Build history of the part. All positions in model axes, mm. A direction names the side the tool comes from. Coordinates: 2 decimals unless noted, no trailing zeros. Write each loop counter-clockwise with the first axis right and the second up, starting at its lowest first coordinate (ties: lowest second). Pieces come first, ordered by that corner, then holes.
```python
from build123d import *

# Parameters (mm, degrees)
SKETCH_1_W          = 20
SKETCH_1_H          = 10
SKETCH_1_W_2        = 18
SKETCH_1_H_2        = 8
EXTRUDE_1_DEPTH     = 30
SKETCH_2_R          = 1.5
CUT_EXTRUDE_1_DEPTH = 20
SKETCH_3_R          = 3.5
CUT_EXTRUDE_2_DEPTH = 5


with BuildPart() as part:
    # 草图1 → 拉伸-薄壁1 (new body)
    with BuildSketch(Plane.XY):
        with Locations((19.212936099, 31.397704236)):
            Rectangle(SKETCH_1_W, SKETCH_1_H)
        with Locations((19.212936099, 31.397704236)):
            Rectangle(SKETCH_1_W_2, SKETCH_1_H_2, mode=Mode.SUBTRACT)
    extrude(amount=EXTRUDE_1_DEPTH)

    # 草图2 → 切除-拉伸1 (cut)
    with BuildSketch(Plane(origin=(29.212936099, 0, 0), x_dir=(0, 0, -1), z_dir=(1, 0, 0))):
        with Locations((-23, 31.397704236)):
            Circle(SKETCH_2_R)
        with Locations((-6, 31.397704236)):
            Circle(SKETCH_2_R)
    extrude(amount=-CUT_EXTRUDE_1_DEPTH, mode=Mode.SUBTRACT)

    # 草图3 → 切除-拉伸2 (cut)
    with BuildSketch(Plane(origin=(29.212936099, 0, 0), x_dir=(0, 0, -1), z_dir=(1, 0, 0))):
        with Locations((-23, 31.397704236)):
            Circle(SKETCH_3_R)
        with Locations((-6, 31.397704236)):
            Circle(SKETCH_3_R)
    extrude(amount=-CUT_EXTRUDE_2_DEPTH, mode=Mode.SUBTRACT)


solid = part.part
```
1. Saw through at A-A on z = 6. List the corners of the cut face in (x, y), plus the area to 3 significant figures.
Computed values:
outline: (9.21, 26.4) - (29.21, 26.4) - (29.21, 27.9) - (28.21, 27.9) - (28.21, 27.4) - (10.21, 27.4) - (10.21, 29.9) - (9.21, 29.9) - close; (9.21, 32.9) - (10.21, 32.9) - (10.21, 35.4) - (28.21, 35.4) - (28.21, 34.9) - (29.21, 34.9) - (29.21, 36.4) - (9.21, 36.4) - close
area: 46.0 mm2
2. Probe line 1 along Y through (x, z) = (9.5, 23); line 2 along X through (y, z) = (33.5, 27.75); line 3 along Y through (x, z) = (28.65, 23). List the from-to ranges inside material, lowest first.
Computed values:
line 1: y = 26.4 to 29.9, 32.9 to 36.4
line 2: x = 9.21 to 10.21, 28.21 to 29.21
line 3: y = 26.4 to 27.9, 34.9 to 36.4
3. Mould opens along Y. For faces 1 (the face through (28.213, 31, 15)), 2 (the face through (18, 27, 0)), 3 (the face through (19, 36.398, 15)), 4 (the face through (19, 26.398, 15)) say: +Y half, -Y half, draft (parallel to the pull), parting line (faces both ways), or undercut.
Computed values:
face 1: undercut
face 2: draft
face 3: +Y half
face 4: -Y half
4. Saw through at D-D on z = 27. List the corners of the cut face in (x, y).
Computed values:
outline: (9.21, 26.4) - (29.21, 26.4) - (29.21, 36.4) - (9.21, 36.4) - close; hole (10.21, 27.4) - (28.21, 27.4) - (28.21, 35.4) - (10.21, 35.4) - close
5. Saw through at B-B on x = 16.25. List the corners of the cut face in (y, z).
Computed values:
outline: (26.4, 0) - (27.4, 0) - (27.4, 30) - (26.4, 30) - close; (35.4, 0) - (36.4, 0) - (36.4, 30) - (35.4, 30) - close
6. Flat gauge pins, fed straight in: pin 1 (3 mm diameter, centred on x = 25.5, y = 29, fed in from +Z); pin 2 (5.5 mm diameter, centred on y = 31.4, z = 6, fed in from +X). Where does each tip first touch, or does it go through?
Computed values:
pin 1: passes through
pin 2: stops at x = 10.21
7. 3-axis set-ups, long thin cutter, end or side, ignore diameter. For faces 5 (the face through (19, 35.398, 15)), 6 (the face through (28.72, 28.293, 21.385)), 7 (the face through (18, 27, 30)): which of +Z, -Z, +X, -X, +Y, -Y reach the whole face in a straight line?
Computed values:
face 5: +Z, -Z
face 6: +X
face 7: +Z, +X, -X, +Y, -Y
8. Saw through at C-C on y = 32. List the corners of the cut face in (x, z).
Computed values:
outline: (9.21, 0) - (10.21, 0) - (10.21, 4.63) - (9.21, 4.63) - close; (9.21, 7.37) - (10.21, 7.37) - (10.21, 21.63) - (9.21, 21.63) - close; (9.21, 24.37) - (10.21, 24.37) - (10.21, 30) - (9.21, 30) - close; (28.21, 0) - (29.21, 0) - (29.21, 2.55) - (28.21, 2.55) - close; (28.21, 9.45) - (29.21, 9.45) - (29.21, 19.55) - (28.21, 19.55) - close; (28.21, 26.45) - (29.21, 26.45) - (29.21, 30) - (28.21, 30) - close
